Design review of the part built by this model. Coordinates are the model's own, in mm. A direction names the side the tool comes from. Round coordinates to 2 decimals unless told otherwise and drop trailing zeros. Order: outer loops, then holes, each group sorted by start corner. A loop starts at its lowest first (then second) coordinate and runs counter-clockwise, first axis right, second up. Notation, with made-up numbers: (0.25, 56) - (30.25, 56) arc R12 cw to (30.25, 67) - close; hole circle Ø1 at (36, 37). An arc over 180 degrees is marked (long way). Use CSV: the item, a comma, the result in double quotes.
from build123d import *

# Parameters (mm, degrees)
SKETCH1_R               = 1.651
BOSS_EXTRUDE1_DEPTH     = 6.985
SKETCH3_R               = 2.286
BOSS_EXTRUDE2_DEPTH     = 2.54
CUT_EXTRUDE3_DEPTH      = 2.54
CUT_EXTRUDE3_DEPTH_BACK = 2.54
FILLET1_R               = 0.508


with BuildPart() as part:
    # Sketch1 → Boss-Extrude1 (new body)
    with BuildSketch(Plane.XY):
        Circle(SKETCH1_R)
    extrude(amount=BOSS_EXTRUDE1_DEPTH)

    # Sketch3 → Boss-Extrude2 (add)
    with BuildSketch(Plane.XY.offset(6.985)):
        Circle(SKETCH3_R)
    extrude(amount=BOSS_EXTRUDE2_DEPTH)

    # Sketch2 → Cut-Extrude3 (cut, two sides)
    with BuildSketch(Plane.XY.offset(6.985)) as cut_extrude3_sk:
        with BuildLine():
            Line((-0.889, 0), (-0.889, -0.381))
            Line((-0.889, -0.381), (0.7112, -0.381))
            Line((0.7112, -0.381), (0.889, -0.381))
            Line((0.889, -0.381), (0.889, 0))
            ThreePointArc((0.889, 0), (0, 0.889), (-0.889, 0))
        make_face()
    extrude(amount=CUT_EXTRUDE3_DEPTH, mode=Mode.SUBTRACT)
    extrude(cut_extrude3_sk.sketch, amount=-CUT_EXTRUDE3_DEPTH_BACK, mode=Mode.SUBTRACT)

    # Fillet1
    fillet1_edges = [part.edges().sort_by_distance(p)[0] for p in [
        (-1.651, 0, 6.985),
    ]]
    fillet(fillet1_edges, radius=FILLET1_R)


solid = part.part
1) We need section A-A (x = 0). Give the boundary of the cut face in (y, z) (3 decimals), then the cut area to 3 significant figures.
Data:
outline,"(-2.286, 6.985) - (-2.159, 6.985) arc R0.508 cw to (-1.651, 6.477) - (-1.651, 0) - (1.651, 0) - (1.651, 6.477) arc R0.508 cw to (2.159, 6.985) - (2.286, 6.985) - (2.286, 9.525) - (0.889, 9.525) - (0.889, 4.445) - (-0.381, 4.445) - (-0.381, 9.525) - (-2.286, 9.525) - close"
area,"28.3 mm2"
2) Insertion check: pin 1 Ø2 at (y, z) = (0.5, 2.5) entering from -X; pin 2 Ø0.9 at (x, z) = (0, 6) entering from +Y. Each pin has a flat end and moves straight along its axis. Give the tip position at first contact, or say it passes through.
Data:
pin 1,"stops at x = -1.65"
pin 2,"stops at y = 1.65"
3) To check wall thickness, follow L1, parallel to Y at x = -0.15, z = 8; L2, parallel to Y at x = 0.65, z = 5.75; L3, parallel to Y at x = 0.1, z = 2. State the ranges of each line that lie inside material, in increasing order. Write a range as from..to.
Data:
L1,"y = -2.28..-0.38, 0.88..2.28"
L2,"y = -1.52..-0.38, 0.61..1.52"
L3,"y = -1.65..1.65"
4) We need section B-B (z = 8.75). Give the boundary of the cut face in (x, y), then the cut area to 3 significant figures.
Data:
outline,"circle Ø4.57 at (0, 0); hole (-0.89, -0.38) - (0.89, -0.38) - (0.89, 0) arc R0.89 ccw to (-0.89, 0) - close"
area,"14.5 mm2"
5) We need section C-C (z = 1.25). Give the boundary of the cut face in (x, y), then the cut area to 3 significant figures.
Data:
outline,"circle Ø3.3 at (0, 0)"
area,"8.56 mm2"
6) The part is to be moulded in two halves that separate along Y. For faces 1 (the face through (0, -1, 9.525)), 2 (the face through (1.525, -0.632, 3.193)), 3 (the face through (0, -0.381, 7)), say which applies: +Y half, -Y half, draft (parallel to the pull), parting line (faces both ways), or undercut.
Data:
face 1,"draft"
face 2,"parting line"
face 3,"undercut"
7) We need section D-D (z = 4.75). Give the boundary of the cut face in (x, y).
Data:
outline,"circle Ø3.3 at (0, 0); hole (-0.89, -0.38) - (0.89, -0.38) - (0.89, 0) arc R0.89 ccw to (-0.89, 0) - close"
8) For faces 4 (the face through (0, 0, 0)), 5 (the face through (0.02, 0.89, 6.95)), list the 3-axis set-ups (+Z, -Z, +X, -X, +Y, -Y) from which the entire face can be reached by the end or side of a thin tool; tool diameter is ignored.
Data:
face 4,"-Z, +X, -X, +Y, -Y"
face 5,"+Z"
